from build123d import *

# Parameters (mm, degrees)
SKETCH1_W           = 12
SKETCH1_H           = 7
BOSS_EXTRUDE1_DEPTH = 36.5
SKETCH3_W           = 12
SKETCH3_H           = 5
BOSS_EXTRUDE2_DEPTH = 11.5
FILLET1_R           = 2
FILLET2_R           = 5
CUT_EXTRUDE1_REACH  = 14
SKETCH7_R           = 1.5


with BuildPart() as part:
    # Sketch1 → Boss-Extrude1 (new body, symmetric)
    with BuildSketch(Plane(origin=(0, 0, 0), x_dir=(1, 0, 0), z_dir=(0, 1, 0))):
        Rectangle(SKETCH1_W, SKETCH1_H)
    extrude(amount=BOSS_EXTRUDE1_DEPTH, both=True)

    # Sketch3 → Boss-Extrude2 (add, symmetric)
    with BuildSketch(Plane.XY):
        with Locations((0, -34)):
            Rectangle(SKETCH3_W, SKETCH3_H)
    extrude(amount=BOSS_EXTRUDE2_DEPTH, both=True)

    # Fillet1
    fillet1_edges = [part.edges().sort_by_distance(p)[0] for p in [
        (-6, -34, -11.5),
        (6, -34, -11.5),
        (-6, -34, 11.5),
        (6, -34, 11.5),
    ]]
    fillet(fillet1_edges, radius=FILLET1_R)

    # Sketch6 → CBORE for M3 Hex Socket Head Cap Screw1 (revolve, cut)
    with BuildSketch(Plane(origin=(0, -31.5, -7.3), x_dir=(0, 0, 1), z_dir=(1, 0, 0))):
        Polygon((0, 0), (0, 5), (1.7, 5), (1.7, 3.4), (3.25, 3.4), (3.25, 0.025), (3.275, 0), align=None)
    cbore_for_m3_hex_socket_head_cap_screw1 = revolve(axis=Axis((0, -25.15, -7.3), (0, -1, 0)), mode=Mode.SUBTRACT)

    # Mirror1: CBORE for M3 Hex Socket Head Cap Screw1 across plane
    add(cbore_for_m3_hex_socket_head_cap_screw1.mirror(Plane.XY), mode=Mode.SUBTRACT)

    # Fillet2
    fillet2_edges = [part.edges().sort_by_distance(p)[0] for p in [
        (-6, 36.5, 0),
    ]]
    fillet(fillet2_edges, radius=FILLET2_R)

    # Sketch7 → Cut-Extrude1 (cut, up to next)
    with BuildSketch(Plane(origin=(6, 0, 0), x_dir=(0, 0, -1), z_dir=(1, 0, 0)), mode=Mode.PRIVATE) as cut_extrude1_sk1:
        with Locations((-0.4, 31.5)):
            Circle(SKETCH7_R)
    cut_extrude1_tool1 = extrude(cut_extrude1_sk1.sketch, amount=-CUT_EXTRUDE1_REACH, mode=Mode.PRIVATE) & part.part
    add(cut_extrude1_tool1.solids().sort_by_distance((6, 31.5, 0.4))[0], mode=Mode.SUBTRACT)
    # Sketch7 → Cut-Extrude1 (cut, up to next)
    with BuildSketch(Plane(origin=(6, 0, 0), x_dir=(0, 0, -1), z_dir=(1, 0, 0)), mode=Mode.PRIVATE) as cut_extrude1_sk2:
        with Locations((-0.4, 21.5)):
            Circle(SKETCH7_R)
    cut_extrude1_tool2 = extrude(cut_extrude1_sk2.sketch, amount=-CUT_EXTRUDE1_REACH, mode=Mode.PRIVATE) & part.part
    add(cut_extrude1_tool2.solids().sort_by_distance((6, 21.5, 0.4))[0], mode=Mode.SUBTRACT)


solid = part.part
Work out the finished part from the listing and answer in its coordinate system (mm). A direction names the side the tool comes from. Coordinates: 2 decimals unless noted, no trailing zeros. Write each loop counter-clockwise with the first axis right and the second up, starting at its lowest first coordinate (ties: lowest second). Pieces come first, ordered by that corner, then holes.
1. For faces 1 (the cylindrical face through (-0.143, -33.189, -10.547)), 2 (the flat face through (-3, -31.5, -9)), 3 (the flat face through (-6, -11, 0)), determine the directions among +Z, -Z, +X, -X, +Y, -Y from which every point of the face is accessible in a straight line to the end or side of a thin tool.
Results list:
face 1: +Y
face 2: -Z, +X, -X, +Y
face 3: +Z, -Z, -X, +Y, -Y
2. Flat-ended cylindrical pins translate along their axes: pin 1 (5 mm diameter, centred on x = 0, z = 8, fed in from +Y); pin 2 (5 mm diameter, centred on x = -1.5, y = -4.5, fed in from +Z); pin 3 (6.5 mm diameter, centred on x = 2.5, z = 7, fed in from +Y). Find the tip coordinate at first contact, or state that the pin passes through.
Results list:
pin 1: stops at y = -34.9
pin 2: stops at z = 3.5
pin 3: stops at y = -31.5
3. The part is cut by section C-C, the plane x = 5.25. Write down the section's boundary in (y, z).
Results list:
outline: (-36.5, -11.06) - (-31.5, -11.06) - (-31.5, -3.5) - (36.5, -3.5) - (36.5, 3.5) - (-31.5, 3.5) - (-31.5, 11.06) - (-36.5, 11.06) - close; hole circle Ø3 at (21.5, 0.4); hole circle Ø3 at (31.5, 0.4)
4. The part is cut by section D-D, the plane y = -10.5. Write down the section's boundary in (x, z).
Results list:
outline: (-6, -3.5) - (6, -3.5) - (6, 3.5) - (-6, 3.5) - close
5. Consider line 1 along Y through (x, z) = (-0.25, 0.4); line 2 along Z through (x, y) = (0, -33.5); line 3 along Y through (x, z) = (3, 1). Determine where each line is inside the solid, lowest interval first.
Results list:
line 1: y = -36.5 to 20, 23 to 30, 33 to 36.5
line 2: z = -11.5 to -10.55, -4.05 to 4.05, 10.55 to 11.5
line 3: y = -36.5 to 20.13, 22.87 to 30.13, 32.87 to 36.5
6. The part is cut by section B-B, the plane z = 0.5. Write down the section's boundary in (x, y), and give its area (3 significant figures).
Results list:
outline: (-6, -36.5) - (6, -36.5) - (6, 20) - (-6, 20) - close; (-6, 23) - (6, 23) - (6, 30) - (-6, 30) - close; (-5.77, 33) - (6, 33) - (6, 36.5) - (-1, 36.5) arc R5 ccw to start
area: 799 mm2
7. The part is cut by section A-A, the plane y = 21.5. Write down the section's boundary in (x, z).
Results list:
outline: (-6, -3.5) - (6, -3.5) - (6, -1.1) - (-6, -1.1) - close; (-6, 1.9) - (6, 1.9) - (6, 3.5) - (-6, 3.5) - close
8. For a pull along Z with two mould halves and no side action, classify faces 4 (the flat face through (0, -36.5, 0)), 5 (the flat face through (0, 3, 3.5)), 6 (the cylindrical face through (0, -36, 9)), 7 (the flat face through (0, -34, -11.5)) as +Z half, -Z half, draft (parallel to the pull), parting line (faces both ways), or undercut.
Results list:
face 4: draft
face 5: +Z half
face 6: undercut
face 7: -Z half
